```python
from build123d import *

# Parameters (mm, degrees)
EXTRUDE_1_DEPTH     = 6
SKETCH_2_R          = 16.15
CUT_EXTRUDE_1_DEPTH = 4.5
SKETCH_3_R          = 14.85
CUT_EXTRUDE_2_DEPTH = 68.731085921
CHAMFER_1_SIZE      = 1
CHAMFER_1_SIZE2     = 0.900404044
SKETCH_4_W          = 37
SKETCH_4_H          = 6
EXTRUDE_2_DEPTH     = 6.5
SKETCH_5_W          = 14.3
SKETCH_5_H          = 2.8
CUT_EXTRUDE_3_DEPTH = 1.5
SKETCH_6_W          = 11.35
SKETCH_6_H          = 3
EXTRUDE_3_DEPTH     = 28
SKETCH_7_R          = 1.15
CUT_EXTRUDE_4_DEPTH = 69.727723664
CUT_EXTRUDE_5_REACH = 70.728
SKETCH_8_R          = 2.1
CUT_EXTRUDE_START   = -3
SKETCH_9_R          = 10.75
SKETCH_9_W          = 37
SKETCH_9_H          = 9.5
CUT_EXTRUDE_6_DEPTH = 3
CUT_EXTRUDE_7_REACH = 70.728
SKETCH_10_R         = 1.6
CHAMFER_2_SIZE      = 1
CHAMFER_2_SIZE2     = 0.900404044


with BuildPart() as part:
    # 스케치1 → 보스-돌출1 (new body)
    with BuildSketch(Plane(origin=(0, 0, 0), x_dir=(1, 0, 0), z_dir=(0, 1, 0))):
        with BuildLine():
            Line((-18.5, 0), (-18.5, -65))
            Line((-18.5, -65), (18.5, -65))
            Line((18.5, -65), (18.5, 0))
            ThreePointArc((18.5, 0), (0, 18.5), (-18.5, 0))
        make_face()
    extrude(amount=EXTRUDE_1_DEPTH)

    # 스케치2 → 컷-돌출1 (cut)
    with BuildSketch(Plane(origin=(0, 6, 0), x_dir=(1, 0, 0), z_dir=(0, 1, 0))):
        with Locations(Location((0, 0, 0), (0, 0, 270))):
            Circle(SKETCH_2_R)
    extrude(amount=-CUT_EXTRUDE_1_DEPTH, mode=Mode.SUBTRACT)

    # 스케치3 → 컷-돌출2 (cut, through all)
    with BuildSketch(Plane(origin=(0, 1.5, 0), x_dir=(1, 0, 0), z_dir=(0, 1, 0))):
        with Locations(Location((0, 0, 0), (0, 0, 270))):
            Circle(SKETCH_3_R)
    extrude(amount=-CUT_EXTRUDE_2_DEPTH, mode=Mode.SUBTRACT)

    # 모따기1
    chamfer_1_edges = [part.edges().sort_by_distance(p)[0] for p in [
        (0, 6, -16.15),
    ]]
    chamfer_1_side = [part.faces().sort_by_distance(p)[0] for p in [
        (0, 3.75, -16.15),
    ]]
    chamfer(chamfer_1_edges, length=CHAMFER_1_SIZE, length2=CHAMFER_1_SIZE2, reference=chamfer_1_side[0])

    # 스케치4 → 보스-돌출2 (add)
    with BuildSketch(Plane.XZ):
        with Locations((0, 36)):
            Rectangle(SKETCH_4_W, SKETCH_4_H)
        with BuildLine():
            Line((-18.5, 16.5), (-10.5, 16.5))
            Line((-10.5, 16.5), (-10.5, 13.369741957))
            ThreePointArc((-10.5, 13.369741957), (-12.02081528, 12.02081528), (-13.369741957, 10.5))
            Line((-13.369741957, 10.5), (-18.5, 10.5))
            Line((-18.5, 10.5), (-18.5, 16.5))
        make_face()
        with BuildLine():
            Line((18.5, 16.5), (10.5, 16.5))
            Line((10.5, 16.5), (10.5, 13.369741957))
            ThreePointArc((10.5, 13.369741957), (12.02081528, 12.02081528), (13.369741957, 10.5))
            Line((13.369741957, 10.5), (18.5, 10.5))
            Line((18.5, 10.5), (18.5, 16.5))
        make_face()
    extrude(amount=EXTRUDE_2_DEPTH)

    # 스케치5 → 컷-돌출3 (cut)
    with BuildSketch(Plane.XZ.offset(6.5)):
        with Locations((0, 34.4)):
            Rectangle(SKETCH_5_W, SKETCH_5_H)
    extrude(amount=-CUT_EXTRUDE_3_DEPTH, mode=Mode.SUBTRACT)

    # 스케치6 → 보스-돌출3 (add)
    with BuildSketch(Plane(origin=(0, 0, 33), x_dir=(-1, 0, 0), z_dir=(0, 0, -1))):
        with Locations((-12.825, -5)):
            Rectangle(SKETCH_6_W, SKETCH_6_H)
        with Locations((12.825, -5)):
            Rectangle(SKETCH_6_W, SKETCH_6_H)
    extrude(amount=EXTRUDE_3_DEPTH)

    # 스케치7 → 컷-돌출4 (cut, through all)
    with BuildSketch(Plane.XZ.offset(6.5)):
        with Locations(Location((-10.25, 29, 0), (0, 0, 270))):
            Circle(SKETCH_7_R)
        with Locations(Location((10.25, 29, 0), (0, 0, 270))):
            Circle(SKETCH_7_R)
        with Locations(Location((-10.25, 8.5, 0), (0, 0, 270))):
            Circle(SKETCH_7_R)
        with Locations(Location((10.25, 8.5, 0), (0, 0, 270))):
            Circle(SKETCH_7_R)
    extrude(amount=-CUT_EXTRUDE_4_DEPTH, mode=Mode.SUBTRACT)

    # 스케치8 → 컷-돌출5 (cut, up to next)
    with BuildSketch(Plane(origin=(0, 6, 0), x_dir=(1, 0, 0), z_dir=(0, 1, 0)), mode=Mode.PRIVATE) as cut_extrude_5_sk1:
        with Locations(Location((-10.25, -29, 0), (0, 0, 270))):
            Circle(SKETCH_8_R)
    cut_extrude_5_tool1 = extrude(cut_extrude_5_sk1.sketch, amount=-CUT_EXTRUDE_5_REACH, mode=Mode.PRIVATE) & part.part
    # 스케치8 → 컷-돌출5 (cut, up to next)
    with BuildSketch(Plane(origin=(0, 6, 0), x_dir=(1, 0, 0), z_dir=(0, 1, 0)), mode=Mode.PRIVATE) as cut_extrude_5_sk2:
        with Locations(Location((10.25, -29, 0), (0, 0, 270))):
            Circle(SKETCH_8_R)
    cut_extrude_5_tool2 = extrude(cut_extrude_5_sk2.sketch, amount=-CUT_EXTRUDE_5_REACH, mode=Mode.PRIVATE) & part.part
    add(cut_extrude_5_tool1.solids().sort_by_distance((-10.25, 6, 29))[0], mode=Mode.SUBTRACT)
    add(cut_extrude_5_tool2.solids().sort_by_distance((10.25, 6, 29))[0], mode=Mode.SUBTRACT)

    # 스케치9 → 컷-돌출6 (cut)
    with BuildSketch(Plane.XZ.offset(6.5).offset(CUT_EXTRUDE_START)):
        Circle(SKETCH_9_R)
        with Locations((0, 21.25)):
            Rectangle(SKETCH_9_W, SKETCH_9_H)
    extrude(amount=CUT_EXTRUDE_6_DEPTH, mode=Mode.SUBTRACT)

    # 스케치10 → 컷-돌출7 (cut, up to next)
    with BuildSketch(Plane(origin=(0, 6, 0), x_dir=(1, 0, 0), z_dir=(0, 1, 0)), mode=Mode.PRIVATE) as cut_extrude_7_sk1:
        with Locations(Location((-15.5, -52, 0), (0, 0, 270))):
            Circle(SKETCH_10_R)
    cut_extrude_7_tool1 = extrude(cut_extrude_7_sk1.sketch, amount=-CUT_EXTRUDE_7_REACH, mode=Mode.PRIVATE) & part.part
    # 스케치10 → 컷-돌출7 (cut, up to next)
    with BuildSketch(Plane(origin=(0, 6, 0), x_dir=(1, 0, 0), z_dir=(0, 1, 0)), mode=Mode.PRIVATE) as cut_extrude_7_sk2:
        with Locations(Location((15.5, -52, 0), (0, 0, 270))):
            Circle(SKETCH_10_R)
    cut_extrude_7_tool2 = extrude(cut_extrude_7_sk2.sketch, amount=-CUT_EXTRUDE_7_REACH, mode=Mode.PRIVATE) & part.part
    # 스케치10 → 컷-돌출7 (cut, up to next)
    with BuildSketch(Plane(origin=(0, 6, 0), x_dir=(1, 0, 0), z_dir=(0, 1, 0)), mode=Mode.PRIVATE) as cut_extrude_7_sk3:
        with Locations(Location((15.5, -62, 0), (0, 0, 270))):
            Circle(SKETCH_10_R)
    cut_extrude_7_tool3 = extrude(cut_extrude_7_sk3.sketch, amount=-CUT_EXTRUDE_7_REACH, mode=Mode.PRIVATE) & part.part
    # 스케치10 → 컷-돌출7 (cut, up to next)
    with BuildSketch(Plane(origin=(0, 6, 0), x_dir=(1, 0, 0), z_dir=(0, 1, 0)), mode=Mode.PRIVATE) as cut_extrude_7_sk4:
        with Locations(Location((-15.5, -62, 0), (0, 0, 270))):
            Circle(SKETCH_10_R)
    cut_extrude_7_tool4 = extrude(cut_extrude_7_sk4.sketch, amount=-CUT_EXTRUDE_7_REACH, mode=Mode.PRIVATE) & part.part
    add(cut_extrude_7_tool1.solids().sort_by_distance((-15.5, 6, 52))[0], mode=Mode.SUBTRACT)
    add(cut_extrude_7_tool2.solids().sort_by_distance((15.5, 6, 52))[0], mode=Mode.SUBTRACT)
    add(cut_extrude_7_tool3.solids().sort_by_distance((15.5, 6, 62))[0], mode=Mode.SUBTRACT)
    add(cut_extrude_7_tool4.solids().sort_by_distance((-15.5, 6, 62))[0], mode=Mode.SUBTRACT)

    # 모따기2
    chamfer_2_edges = [part.edges().sort_by_distance(p)[0] for p in [
        (-15.5, 0, 60.4),
        (15.5, 0, 60.4),
        (15.5, 0, 50.4),
        (-15.5, 0, 50.4),
    ]]
    chamfer_2_side = [part.faces().sort_by_distance(p)[0] for p in [
        (0, 0, 51.827011897),
    ]]
    chamfer(chamfer_2_edges, length=CHAMFER_2_SIZE, length2=CHAMFER_2_SIZE2, reference=chamfer_2_side[0])


solid = part.part
```
Geometry check sheet. Reference: the model listing, model coordinates, mm. A direction names the side the tool comes from. Give positions to 0.01 mm unless a question says otherwise; leave off trailing zeros. Order: outer loops, then holes, each group sorted by start corner. A loop starts at its lowest first (then second) coordinate and runs counter-clockwise, first axis right, second up. Notation, with made-up numbers: (48.5, 85) - (82.5, 85) arc R24 ccw to (82.5, 119) - close; hole circle Ø7 at (53.25, 46). An arc over 180 degrees is marked (long way). Answer in a Markdown table with one row per item. Add a question column.
Q1. Cross-section at C-C, the plane y = 3.25. Enter the section's corners in (x, z), then the cut area to 3 significant figures.
Q2. Tool access check on faces 5 (the flat face through (-14, -3, 16.5)), 6 (the flat face through (10.5, -2, 15)), 7 (the flat face through (-16, -2, 10.5)), 8 (the cylindrical face through (-15.766, 3.274, -3.501)), 9 (the cylindrical face through (8.486, -4.979, 6.599)). Record the directions out of +Z, -Z, +X, -X, +Y, -Y that give a thin tool (end or side, any length) a straight path to the whole face; none if there is none.
Q3. Cross-section at A-A, the plane y = -2.5. Enter the section's corners in (x, z).
Q4. Gauge pin test, flat ends, axial feed: pin 1 (1 mm diameter, centred on x = 6, z = 43, fed in from -Y); pin 2 (1.6 mm diameter, centred on x = 3, y = -5.5, fed in from -Z); pin 3 (2 mm diameter, centred on x = 11, z = 29.5, fed in from +Y). Record the tip position at first contact, or that the pin passes through.
Q5. Material ranges on probe 1 along X at (y, z) = (4.1, 52); probe 2 along X at (y, z) = (3.2, 29); probe 3 along Z at (x, y) = (-14, -4.75), recorded low to high. Write a range as from..to.
Q6. Mould release check, pull along X, two halves, no side actions. Record for faces 1 (the flat face through (-7.15, -5, 30)), 2 (the flat face through (-14, -5, 5)), 3 (the cylindrical face through (0.407, 2.958, -18.496)), 4 (the flat face through (-10.5, -2, 15)): pulls with the +X half, pulls with the -X half, needs draft (parallel to the pull), parting line crosses it, or undercut.
Q7. Cross-section at D-D, the plane x = 0. Enter the section's corners in (y, z), then the cut area to 3 significant figures.
Q8. Cross-section at B-B, the plane z = 62. Enter the section's corners in (x, y).
Check values:
| question | item | result |
|---|---|---|
| 1 | outline | (-18.5, 0) arc R18.5 ccw to (18.5, 0) - (18.5, 65) - (-18.5, 65) - close; hole circle Ø3.2 at (-15.5, 52); hole circle Ø3.2 at (-15.5, 62); hole circle Ø32.3 at (0, 0); hole circle Ø4.2 at (-10.25, 29); hole circle Ø4.2 at (10.25, 29); hole circle Ø3.2 at (15.5, 52); hole circle Ø3.2 at (15.5, 62) |
| 1 | area | 2,060 mm^2 |
| 2 | face 5 | +X, -X, -Y |
| 2 | face 6 | -Z |
| 2 | face 7 | -Z, +X, -X |
| 2 | face 8 | +Y |
| 2 | face 9 | -Z, +Y, -Y |
| 3 | outline | (-18.5, 10.5) - (-13.37, 10.5) arc R17 cw to (-10.5, 13.37) - (-10.5, 16.5) - (-18.5, 16.5) - close; (-18.5, 33) - (18.5, 33) - (18.5, 39) - (-18.5, 39) - close; (10.5, 13.37) arc R17 cw to (13.37, 10.5) - (18.5, 10.5) - (18.5, 16.5) - (10.5, 16.5) - close |
| 4 | pin 1 | stops at y = 0 |
| 4 | pin 2 | stops at z = 33 |
| 4 | pin 3 | stops at y = -3.5 |
| 5 | probe 1 | x = -18.5..-17.1, -13.9..13.9, 17.1..18.5 |
| 5 | probe 2 | x = -18.5..-12.35, -8.15..8.15, 12.35..18.5 |
| 5 | probe 3 | z = 5..16.5, 26..39 |
| 6 | face 1 | undercut |
| 6 | face 2 | needs draft |
| 6 | face 3 | parting line crosses it |
| 6 | face 4 | undercut |
| 7 | outline | (-6.5, 35.8) - (-5, 35.8) - (-5, 33) - (0, 33) - (0, 14.85) - (1.5, 14.85) - (1.5, 16.15) - (5, 16.15) - (6, 17.05) - (6, 65) - (0, 65) - (0, 39) - (-6.5, 39) - close; (0, -18.5) - (6, -18.5) - (6, -17.05) - (5, -16.15) - (1.5, -16.15) - (1.5, -14.85) - (0, -14.85) - close |
| 7 | area | 345 mm^2 |
| 8 | outline | (-18.5, 0) - (-18.1, 0) - (-17.1, 0.9) - (-17.1, 6) - (-18.5, 6) - close; (-13.9, 0.9) - (-12.9, 0) - (12.9, 0) - (13.9, 0.9) - (13.9, 6) - (-13.9, 6) - close; (17.1, 0.9) - (18.1, 0) - (18.5, 0) - (18.5, 6) - (17.1, 6) - close |
